```python
from build123d import *

# Parameters (mm, degrees)
SKETCH1_R           = 6.5
SKETCH1_R_2         = 6
BOSS_EXTRUDE1_DEPTH = 10
BOSS_EXTRUDE2_START = 0.5
SKETCH2_R           = 6.5
BOSS_EXTRUDE2_DEPTH = 0.5
SKETCH3_R           = 6.5
BOSS_EXTRUDE3_DEPTH = 0.5
CHAMFER1_SIZE       = 0.5
CHAMFER1_SIZE2      = 0.482844387
SKETCH4_W           = 2.9
SKETCH4_H           = 3.6
CUT_EXTRUDE1_DEPTH  = 1
FILLET1_R           = 0.1
FILLET2_R           = 0.3


with BuildPart() as part:
    # Sketch1 → Boss-Extrude1 (new body)
    with BuildSketch(Plane.XY):
        Circle(SKETCH1_R)
        Circle(SKETCH1_R_2, mode=Mode.SUBTRACT)
    extrude(amount=BOSS_EXTRUDE1_DEPTH)

    # Sketch2 → Boss-Extrude2 (add)
    with BuildSketch(Plane(origin=(0, 0, 0), x_dir=(-1, 0, 0), z_dir=(0, 0, -1)).offset(BOSS_EXTRUDE2_START)):
        Circle(SKETCH2_R)
    extrude(amount=-BOSS_EXTRUDE2_DEPTH)

    # Sketch3 → Boss-Extrude3 (add)
    with BuildSketch(Plane.XY.offset(10)):
        with Locations(Location((0, 0, 0), (0, 0, 180))):
            Circle(SKETCH3_R)
        Polygon((-2.2, 3.7), (-2.2, -3.7), (2.2, -4.1), (2.2, 4.1), align=None, mode=Mode.SUBTRACT)
    extrude(amount=BOSS_EXTRUDE3_DEPTH)

    # Chamfer1
    chamfer1_edges = [part.edges().sort_by_distance(p)[0] for p in [
        (0, -3.9, 10.5),
        (2.2, 0, 10.5),
        (0, 3.9, 10.5),
        (-2.2, 0, 10.5),
    ]]
    chamfer1_side = [part.faces().sort_by_distance(p)[0] for p in [
        (6.316152237, 0, 10.5),
    ]]
    chamfer(chamfer1_edges, length=CHAMFER1_SIZE, length2=CHAMFER1_SIZE2, reference=chamfer1_side[0])

    # Sketch4 → Cut-Extrude1 (cut)
    with BuildSketch(Plane(origin=(0, 0, -0.5), x_dir=(-1, 0, 0), z_dir=(0, 0, -1))):
        Rectangle(SKETCH4_W, SKETCH4_H)
    extrude(amount=-CUT_EXTRUDE1_DEPTH, mode=Mode.SUBTRACT)

    # Fillet1
    fillet1_edges = [part.edges().sort_by_distance(p)[0] for p in [
        (-1.45, 1.8, -0.25),
        (-1.45, -1.8, -0.25),
        (1.45, -1.8, -0.25),
        (1.45, 1.8, -0.25),
    ]]
    fillet(fillet1_edges, radius=FILLET1_R)

    # Fillet2
    fillet2_edges = [part.edges().sort_by_distance(p)[0] for p in [
        (6.5, 0, -0.5),
        (6.5, 0, 10.5),
    ]]
    fillet(fillet2_edges, radius=FILLET2_R)


solid = part.part
```
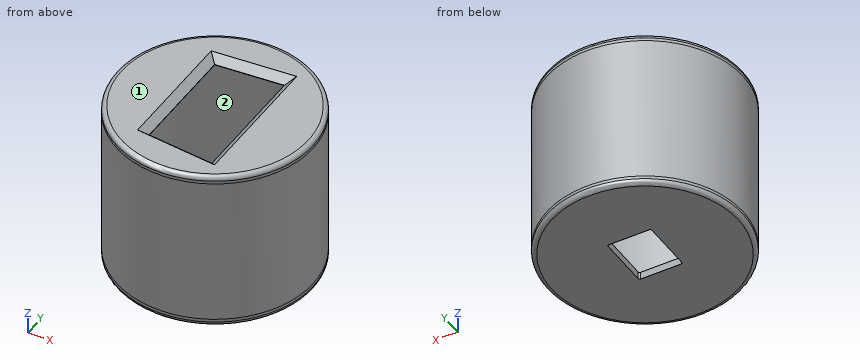
Geometry: final body of the model. Coordinates: model frame, mm. Face numbers are marked on the shaded views. Coordinates: 2 decimals unless noted, no trailing zeros. Order: outer loops, then holes, each group sorted by start corner. A loop starts at its lowest first (then second) coordinate and runs counter-clockwise, first axis right, second up. Notation, with made-up numbers: (60, 59) - (115, 59) arc R18 cw to (115, 94) - close; hole circle Ø2 at (-39.75, -38). An arc over 180 degrees is marked (long way). Return JSON: item names as keys, results as strings. Group by question number.
1. Pin query (flat end, axial travel): pin 1 (6 mm diameter, centred on y = 3.5, z = 8, fed in from +X); pin 2 (6 mm diameter, centred on x = 3.5, z = 8.5, fed in from +Y); pin 3 (3 mm diameter, centred on y = -5, z = 6, fed in from -X). Return the tip coordinate at first contact, or that it passes through.
2. Material intervals for line 1 along Z through (x, y) = (3, -4.5); line 2 along Y through (x, z) = (0, 6); line 3 along X through (y, z) = (4.5, 5.5), sorted ascending. Write a range as [from, to].
3. Pull-direction query (X, two-part tool) for the marked faces 1 and 2; classes: pulls with the +X half, pulls with the -X half, needs draft (parallel to the pull), parting line crosses it, or undercut.
4. Cut plane C-C (z = 0.75). Output: boundary loops of the cut face in (x, y).
Resolved:
{
 "1": {"pin 1": "stops at x = 6.48", "pin 2": "stops at y = 6.48", "pin 3": "stops at x = -5.48"},
 "2": {"line 1": "z = [-0.5, 0], [10, 10.5]", "line 2": "y = [-6.5, -6], [6, 6.5]", "line 3": "x = [-4.69, -3.97], [3.97, 4.69]"},
 "3": {"face 1": "needs draft", "face 2": "undercut"},
 "4": {"outline": "circle Ø13 at (0, 0); hole circle Ø12 at (0, 0)"}
}
